Design review of the part built by this model. Coordinates are the model's own, in mm. Face numbers are marked on the shaded views. A direction names the side the tool comes from. Coordinates: 2 decimals unless noted, no trailing zeros. Write each loop counter-clockwise with the first axis right and the second up, starting at its lowest first coordinate (ties: lowest second). Pieces come first, ordered by that corner, then holes.
Q1. Machinability: for the marked faces 5, 6 and 7, which of the approach directions +Z, -Z, +X, -X, +Y, -Y give a long, thin tool a straight path to every point of the face, cutting with its end or side? Answer none if there is none.
Q2. Add section A-A, the plane x = 14.65. Give the boundary of the cut face in (y, z) (3 decimals).
Q3. Add section D-D, the plane x = 18.75. Give the boundary of the cut face in (y, z).
Q4. Clearance check with flat-ended pins moving along their axes: pin 1 Ø1.9 at (x, y) = (14.65, 2.9) entering from -Z; pin 2 Ø3 at (x, z) = (5, 2.5) entering from +Y. State where each tip first meets the part, or that it passes through.
Q5. To check wall thickness, follow probe 1 along Y at (x, z) = (5.15, 1.5) (3 decimals); probe 2 along X at (y, z) = (2.5, 1.75); probe 3 along Y at (x, z) = (9.25, 2.5). State the ranges of each line that lie inside material, in increasing order.
Q6. Add section B-B, the plane z = 1.75. Give the boundary of the cut face in (x, y) (3 decimals), plus the area to 3 significant figures.
Q7. The part is to be moulded in two halves that separate along X. For the marked faces 1, 2, 3 and 4, say which applies: +X half, -X half, draft (parallel to the pull), parting line (faces both ways), or undercut.
Q8. Add section C-C, the plane y = 2.9. Give the boundary of the cut face in (x, z) (3 decimals).
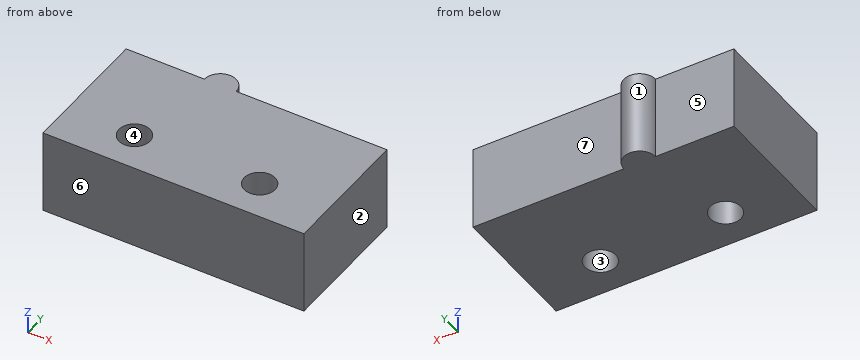
from build123d import *

# Parameters (mm, degrees)
SKETCH1_R           = 1.175
BOSS_EXTRUDE1_DEPTH = 6.4


with BuildPart() as part:
    # Sketch1 → Boss-Extrude1 (new body)
    with BuildSketch(Plane.XY):
        with BuildLine():
            Line((0, 0), (19.8, 0))
            Line((19.8, 0), (19.8, 10.2))
            Line((19.8, 10.2), (8.35, 10.2))
            ThreePointArc((8.35, 10.2), (7.15, 11.4), (5.95, 10.2))
            Line((5.95, 10.2), (0, 10.2))
            Line((0, 10.2), (0, 0))
        make_face()
        with Locations((14.65, 2.9)):
            Circle(SKETCH1_R, mode=Mode.SUBTRACT)
        with Locations((5.15, 2.9)):
            Circle(SKETCH1_R, mode=Mode.SUBTRACT)
    extrude(amount=BOSS_EXTRUDE1_DEPTH)


solid = part.part
Here are the results:
1. face 5: +Z, -Z, -X, +Y
1. face 6: +Z, -Z, +X, -X, -Y
1. face 7: +Z, -Z, +X, +Y
2. outline: (0, 0) - (1.725, 0) - (1.725, 6.4) - (0, 6.4) - close; (4.075, 0) - (10.2, 0) - (10.2, 6.4) - (4.075, 6.4) - close
3. outline: (0, 0) - (10.2, 0) - (10.2, 6.4) - (0, 6.4) - close
4. pin 1: passes through
4. pin 2: stops at y = 11.21
5. probe 1: y = 0 to 1.725, 4.075 to 10.2
5. probe 2: x = 0 to 4.05, 6.25 to 13.55, 15.75 to 19.8
5. probe 3: y = 0 to 10.2
6. outline: (0, 0) - (19.8, 0) - (19.8, 10.2) - (8.35, 10.2) arc R1.2 ccw to (5.95, 10.2) - (0, 10.2) - close; hole circle Ø2.35 at (5.15, 2.9); hole circle Ø2.35 at (14.65, 2.9)
6. area: 196 mm2
7. face 1: parting line
7. face 2: +X half
7. face 3: undercut
7. face 4: undercut
8. outline: (0, 0) - (3.975, 0) - (3.975, 6.4) - (0, 6.4) - close; (6.325, 0) - (13.475, 0) - (13.475, 6.4) - (6.325, 6.4) - close; (15.825, 0) - (19.8, 0) - (19.8, 6.4) - (15.825, 6.4) - close
